from build123d import *

# Parameters (mm, degrees)
SKETCH1_W                                       = 180
SKETCH1_H                                       = 63
BOSS_EXTRUDE1_DEPTH                             = 3
FILLET1_R                                       = 5
SKETCH2_W                                       = 156
SKETCH2_H                                       = 63
BOSS_EXTRUDE2_DEPTH                             = 6
CSK_FOR_M3_FLAT_HEAD_MACHINE_SCREW1_D           = 3.6
CSK_FOR_M3_FLAT_HEAD_MACHINE_SCREW1_DEPTH       = 8
CSK_FOR_M3_FLAT_HEAD_MACHINE_SCREW1_CSINK_D     = 6.8
CSK_FOR_M3_FLAT_HEAD_MACHINE_SCREW1_CSINK_ANGLE = 90
CSK_FOR_M3_FLAT_HEAD_MACHINE_SCREW1_TIP         = 1.081549114
CUT_EXTRUDE1_START                              = -1.5
CUT_EXTRUDE1_DEPTH                              = 1.5
SKETCH6_W                                       = 28
SKETCH6_H                                       = 48
CUT_EXTRUDE2_DEPTH                              = 96.647791402
FILLET2_R                                       = 2
M3_CLEARANCE_HOLE1_D                            = 3.6
M3_CLEARANCE_HOLE1_DEPTH                        = 8
M3_CLEARANCE_HOLE1_TIP                          = 1.081549114
SKETCH15_W                                      = 95
SKETCH15_H                                      = 63
CUT_EXTRUDE3_DEPTH                              = 3
SKETCH18_W                                      = 180
SKETCH18_H                                      = 8
CUT_EXTRUDE8_DEPTH                              = 3
SKETCH21_W                                      = 4
SKETCH21_H                                      = 60
CUT_EXTRUDE10_DEPTH                             = 3
SKETCH22_W                                      = 3
SKETCH22_H                                      = 60
CUT_EXTRUDE11_DEPTH                             = 116.733530146
CUT_EXTRUDE12_DEPTH                             = 0.3
CUT_EXTRUDE13_DEPTH                             = 96.541875636
SKETCH25_W                                      = 114
SKETCH25_H                                      = 50
CUT_EXTRUDE14_DEPTH                             = 96.160548548
SKETCH26_W                                      = 6
SKETCH26_H                                      = 50
CUT_EXTRUDE15_DEPTH                             = 0.3
SKETCH28_W                                      = 156
SKETCH28_H                                      = 3
CUT_EXTRUDE16_DEPTH                             = 3.3


# Read off the part's stored shape, not the designer's step: Cut-Extrude1
with BuildPart() as part:
    # Sketch1 → Boss-Extrude1 (new body)
    with BuildSketch(Plane.XY):
        Rectangle(SKETCH1_W, SKETCH1_H)
    extrude(amount=BOSS_EXTRUDE1_DEPTH)

    # Fillet1
    fillet1_edges = [part.edges().sort_by_distance(p)[0] for p in [
        (90, -31.5, 1.5),
        (-90, -31.5, 1.5),
    ]]
    fillet(fillet1_edges, radius=FILLET1_R)

    # Sketch2 → Boss-Extrude2 (add)
    with BuildSketch(Plane.XY.offset(3)):
        Rectangle(SKETCH2_W, SKETCH2_H)
    extrude(amount=BOSS_EXTRUDE2_DEPTH)

    # CSK for M3 Flat Head Machine Screw1
    with Locations(Plane(origin=(0, 0, 0), x_dir=(-1, 0, 0), z_dir=(0, 0, -1))):
        with Locations((-84, 20), (-84, -20), (84, 20), (84, -20), (-84, 0)):
            CounterSinkHole(CSK_FOR_M3_FLAT_HEAD_MACHINE_SCREW1_D / 2, CSK_FOR_M3_FLAT_HEAD_MACHINE_SCREW1_CSINK_D / 2, depth=CSK_FOR_M3_FLAT_HEAD_MACHINE_SCREW1_DEPTH, counter_sink_angle=CSK_FOR_M3_FLAT_HEAD_MACHINE_SCREW1_CSINK_ANGLE)
            with Locations((0, 0, -(CSK_FOR_M3_FLAT_HEAD_MACHINE_SCREW1_DEPTH + CSK_FOR_M3_FLAT_HEAD_MACHINE_SCREW1_TIP / 2))):  # 118° drill point
                Cone(0, CSK_FOR_M3_FLAT_HEAD_MACHINE_SCREW1_D / 2, CSK_FOR_M3_FLAT_HEAD_MACHINE_SCREW1_TIP, mode=Mode.SUBTRACT)

    # Cut-Extrude1 outline → Cut-Extrude1 (cut)
    with BuildSketch(Plane(origin=(0, 0, 0), x_dir=(-1, 0, 0), z_dir=(0, 0, -1)).offset(CUT_EXTRUDE1_START)):
        with BuildLine():
            Line((77, 30), (47, 30))
            Line((47, 30), (36, 0))
            Line((36, 0), (47, -30))
            Line((47, -30), (77, -30))
            Line((77, -30), (80.604262356, -20.170193575))
            ThreePointArc((80.604262356, -20.170193575), (80.807820526, -18.829534193), (81.519146067, -17.67505618))
            Line((81.519146067, -17.67505618), (88, 0))
            Line((88, 0), (81.519146067, 17.67505618))
            ThreePointArc((81.519146067, 17.67505618), (80.807820526, 18.829534193), (80.604262356, 20.170193575))
            Line((80.604262356, 20.170193575), (77, 30))
        make_face()
    extrude(amount=CUT_EXTRUDE1_DEPTH, mode=Mode.SUBTRACT)

    # Sketch6 → Cut-Extrude2 (cut, through all)
    with BuildSketch(Plane(origin=(0, 0, 1.5), x_dir=(-1, 0, 0), z_dir=(0, 0, -1))):
        with Locations((62, 0)):
            Rectangle(SKETCH6_W, SKETCH6_H)
    extrude(amount=-CUT_EXTRUDE2_DEPTH, mode=Mode.SUBTRACT)

    # Fillet2
    fillet2_edges = [part.edges().sort_by_distance(p)[0] for p in [
        (-36, 0, 0.75),
        (-47, 30, 0.75),
        (-77, 30, 0.75),
        (-88, 0, 0.75),
        (-77, -30, 0.75),
        (-47, -30, 0.75),
    ]]
    fillet(fillet2_edges, radius=FILLET2_R)

    # M3 Clearance Hole1
    with Locations(Plane(origin=(0, 0, 1.5), x_dir=(-1, 0, 0), z_dir=(0, 0, -1))):
        with Locations((42.5, 0), (81.5, 0)):
            Hole(M3_CLEARANCE_HOLE1_D / 2, depth=M3_CLEARANCE_HOLE1_DEPTH)
            with Locations((0, 0, -(M3_CLEARANCE_HOLE1_DEPTH + M3_CLEARANCE_HOLE1_TIP / 2))):  # 118° drill point
                Cone(0, M3_CLEARANCE_HOLE1_D / 2, M3_CLEARANCE_HOLE1_TIP, mode=Mode.SUBTRACT)

    # Sketch15 → Cut-Extrude3 (cut)
    with BuildSketch(Plane.XY.offset(9)):
        with Locations((26.5, 0)):
            Rectangle(SKETCH15_W, SKETCH15_H)
    extrude(amount=-CUT_EXTRUDE3_DEPTH, mode=Mode.SUBTRACT)

    # Sketch18 → Cut-Extrude8 (cut)
    with BuildSketch(Plane(origin=(0, 31.5, 0), x_dir=(1, 0, 0), z_dir=(0, 1, 0))):
        with Locations((0, -7)):
            Rectangle(SKETCH18_W, SKETCH18_H)
    extrude(amount=-CUT_EXTRUDE8_DEPTH, mode=Mode.SUBTRACT)

    # Sketch21 → Cut-Extrude10 (cut)
    with BuildSketch(Plane.XY.offset(9)):
        with Locations((76, -1.5)):
            Rectangle(SKETCH21_W, SKETCH21_H)
    extrude(amount=-CUT_EXTRUDE10_DEPTH, mode=Mode.SUBTRACT)

    # Sketch22 → Cut-Extrude11 (cut, through all)
    with BuildSketch(Plane(origin=(-21, 0, 0), x_dir=(0, 0, -1), z_dir=(1, 0, 0))):
        with Locations((-7.5, -1.5)):
            Rectangle(SKETCH22_W, SKETCH22_H)
    extrude(amount=-CUT_EXTRUDE11_DEPTH, mode=Mode.SUBTRACT)

    # Sketch23 → Cut-Extrude12 (cut)
    with BuildSketch(Plane.XY.offset(3)):
        with BuildLine():
            Line((90, 31.5), (-90, 31.5))
            Line((-90, 31.5), (-90, -26.5))
            ThreePointArc((-90, -26.5), (-88.535533906, -30.035533906), (-85, -31.5))
            Line((-85, -31.5), (-78, -31.5))
            Line((-78, -31.5), (-78, 28.5))
            Line((-78, 28.5), (78, 28.5))
            Line((78, 28.5), (78, -31.5))
            Line((78, -31.5), (85, -31.5))
            ThreePointArc((85, -31.5), (88.535533906, -30.035533906), (90, -26.5))
            Line((90, -26.5), (90, 31.5))
        make_face()
    extrude(amount=-CUT_EXTRUDE12_DEPTH, mode=Mode.SUBTRACT)

    # Sketch24 → Cut-Extrude13 (cut, through all)
    with BuildSketch(Plane(origin=(0, 0, 0), x_dir=(-1, 0, 0), z_dir=(0, 0, -1))):
        with BuildLine():
            Line((90, 31.5), (90, -26.5))
            ThreePointArc((90, -26.5), (88.535533906, -30.035533906), (85, -31.5))
            Line((85, -31.5), (-85, -31.5))
            ThreePointArc((-85, -31.5), (-88.535533906, -30.035533906), (-90, -26.5))
            Line((-90, -26.5), (-90, 31.5))
            Line((-90, 31.5), (90, 31.5))
        make_face()
        with BuildLine():
            Line((-85, -31.2), (85, -31.2))
            ThreePointArc((85, -31.2), (88.323401872, -29.823401872), (89.7, -26.5))
            Line((89.7, -26.5), (89.7, 31.2))
            Line((89.7, 31.2), (-89.7, 31.2))
            Line((-89.7, 31.2), (-89.7, -26.5))
            ThreePointArc((-89.7, -26.5), (-88.323401872, -29.823401872), (-85, -31.2))
        make_face(mode=Mode.SUBTRACT)
    extrude(amount=-CUT_EXTRUDE13_DEPTH, mode=Mode.SUBTRACT)

    # Sketch25 → Cut-Extrude14 (cut, through all)
    with BuildSketch(Plane(origin=(0, 0, 0), x_dir=(-1, 0, 0), z_dir=(0, 0, -1))):
        with Locations((-20.7, -3.2)):
            Rectangle(SKETCH25_W, SKETCH25_H)
    extrude(amount=-CUT_EXTRUDE14_DEPTH, mode=Mode.SUBTRACT)

    # Sketch26 → Cut-Extrude15 (cut)
    with BuildSketch(Plane.ZY.offset(-77.7)):
        with Locations((3, -3.2)):
            Rectangle(SKETCH26_W, SKETCH26_H)
    extrude(amount=-CUT_EXTRUDE15_DEPTH, mode=Mode.SUBTRACT)

    # Sketch28 → Cut-Extrude16 (cut)
    with BuildSketch(Plane.XY.offset(6)):
        with Locations((0, -29.7)):
            Rectangle(SKETCH28_W, SKETCH28_H)
    extrude(amount=-CUT_EXTRUDE16_DEPTH, mode=Mode.SUBTRACT)


solid = part.part
Can you work these out from the model? Positions are in its coordinate system, mm. A direction names the side the tool comes from. Round coordinates to 2 decimals unless told otherwise and drop trailing zeros. Loops run counter-clockwise (first coordinate to the right, second up) from the corner with the lowest first, then second, coordinate; pieces in that order, holes last. Notation, with made-up numbers: (-10.75, 89.5) - (14.25, 89.5) arc R32 cw to (14.25, 118.5) - close; hole circle Ø3 at (-18.75, 17). An arc over 180 degrees is marked (long way). Write item = value, one per line. Start each with the question number.
(1) If we section it at A-A (x = -72.5): Please give me the cut outline in (y, z).
(2) For P1, Ø2, axis at x = -58, z = 5, coming from the +Y side; P2, Ø4.5, axis at x = -84, y = -20, coming from the -Z side; P3, Ø12, axis at x = 24, y = -20.5, coming from the -Z side; P4, Ø1, axis at y = -14, z = 5, coming from the -X side, each with a flat end and sliding along its axis, tell me the tip position at first contact or that it passes through.
(3) If we section it at C-C (x = 31): Please give me the cut outline in (y, z), and give its area (3 significant figures).
(4) If we section it at D-D (y = 14): Please give me the cut outline in (x, z), and give its area (3 significant figures).
(5) If I drill on probe 1 along Y at (x, z) = (84, 2.15); probe 2 along X at (y, z) = (20, 2); probe 3 along X at (y, z) = (11, 2.2), over which ranges is the centre line in solid material (lowest first)? Write a range as [from, to].
(6) If we mould it in two halves opening along X, with no side actions, what happens to faces 5 (the face through (-36.3, -4, 3)), 6 (the face through (-18, 25, 6)), 7 (the face through (78, 25, 4))? For each: released by +X, released by -X, zero draft, split by the parting line, or undercut.
(7) For faces 1 (the face through (-45, 0, 1.5)), 2 (the face through (-57, -28.2, 4)), 3 (the face through (-1, 28.5, 4)), 4 (the face through (-76, 0, 4)), which set-ups out of +Z, -Z, +X, -X, +Y, -Y let a thin tool reach every point of the face, with its end or its side?
(8) If we section it at B-B (z = 3.85): Please give me the cut outline in (x, y).
Ans:
q1.outline = (-31.2, 0) - (-30, 0) - (-30, 1.5) - (-24, 1.5) - (-24, 6) - (-28.2, 6) - (-28.2, 2.7) - (-31.2, 2.7) - close; (24, 1.5) - (30, 1.5) - (30, 0) - (31.2, 0) - (31.2, 2.7) - (28.5, 2.7) - (28.5, 6) - (24, 6) - close
q2.P1 = 28.5
q2.P2 = 1.15
q2.P3 = through
q2.P4 = -78
q3.outline = (-31.2, 0) - (-28.2, 0) - (-28.2, 2.7) - (-31.2, 2.7) - close; (21.8, 0) - (31.2, 0) - (31.2, 2.7) - (28.5, 2.7) - (28.5, 6) - (21.8, 6) - close
q3.area = 55.6 mm²
q4.outline = (-89.7, 0) - (-82.87, 0) - (-82.87, 1.5) - (-76, 1.5) - (-76, 6) - (-78, 6) - (-78, 2.7) - (-89.7, 2.7) - close; (-48, 1.5) - (-41.13, 1.5) - (-41.13, 0) - (-36.3, 0) - (-36.3, 6) - (-48, 6) - close; (78, 0) - (89.7, 0) - (89.7, 2.7) - (78, 2.7) - close
q4.area = 125 mm²
q5.probe_1 = [-31.2, -21.8], [-18.2, -1.8], [1.8, 18.2], [21.8, 31.2]
q5.probe_2 = [-89.7, -85.8], [-82.2, -76], [-48, -36.3], [78, 82.2], [85.8, 89.7]
q5.probe_3 = [-89.7, -76], [-48, -36.3], [78, 89.7]
q6.face_5 = undercut
q6.face_6 = zero draft
q6.face_7 = released by +X
q7.face_1 = -Z
q7.face_2 = +Z, +X, -X, -Y
q7.face_3 = +Z, +X, -X, +Y
q7.face_4 = +Z, -Z
q8.outline = (-78, -28.2) - (-36.3, -28.2) - (-36.3, 21.8) - (78, 21.8) - (78, 28.5) - (-78, 28.5) - close; hole (-76, -24) - (-48, -24) - (-48, 24) - (-76, 24) - close; hole circle Ø3.6 at (-42.5, 0)
